Input: part model. Units: mm. Frame: model coordinates. A direction names the side the tool comes from. Give positions to 0.01 mm unless a question says otherwise; leave off trailing zeros. Order: outer loops, then holes, each group sorted by start corner. A loop starts at its lowest first (then second) coordinate and runs counter-clockwise, first axis right, second up. Notation, with made-up numbers: (6, -20) - (45, -20) arc R17 ccw to (45, -12) - close; hole circle Ø6 at (50, 14.25). An arc over 180 degrees is marked (long way). Use a Markdown table: item, result.
from build123d import *

# Parameters (mm, degrees)
SKETCH1_W                = 12.4
SKETCH1_H                = 5.75
BOSS_EXTRUDE1_DEPTH      = 7
SHELL1_T                 = -0.8
CUT_EXTRUDE1_DEPTH       = 13.4
CUT_EXTRUDE2_REACH       = 7.75
SKETCH4_W                = 0.64
SKETCH4_H                = 0.64
BOSS_EXTRUDE2_DEPTH      = 3.45
BOSS_EXTRUDE2_DEPTH_BACK = 6.75
CHAMFER1_SIZE            = 0.2


with BuildPart() as part:
    # Sketch1 → Boss-Extrude1 (new body)
    with BuildSketch(Plane(origin=(0, 0, 0), x_dir=(1, 0, 0), z_dir=(0, 1, 0))):
        Rectangle(SKETCH1_W, SKETCH1_H)
    extrude(amount=BOSS_EXTRUDE1_DEPTH)

    # Shell1
    shell1_openings = [part.faces().sort_by_distance(p)[0] for p in [
        (0, 7, 0),
    ]]
    offset(amount=SHELL1_T, openings=shell1_openings, kind=Kind.INTERSECTION)

    # Sketch2 → Cut-Extrude1 (cut, through all)
    with BuildSketch(Plane(origin=(6.2, 0, 0), x_dir=(0, 0, -1), z_dir=(1, 0, 0))):
        with BuildLine():
            Line((-1.19301282, 7), (-1.19301282, 4.379603984))
            ThreePointArc((-1.19301282, 4.379603984), (-1.72610374, 4.600417472), (-1.946917229, 5.133508392))
            Line((-1.946917229, 5.133508392), (-1.946917229, 7))
            Line((-1.946917229, 7), (-1.19301282, 7))
        make_face()
    extrude(amount=-CUT_EXTRUDE1_DEPTH, mode=Mode.SUBTRACT)

    # Sketch3 → Cut-Extrude2 (cut, up to next)
    with BuildSketch(Plane.XY.offset(2.875), mode=Mode.PRIVATE) as cut_extrude2_sk1:
        with BuildLine():
            Line((-4.2, 7), (-4.2, 6.728922615))
            Line((-4.2, 6.728922615), (-4.2, 5.166308225))
            ThreePointArc((-4.2, 5.166308225), (-3.946286554, 4.553789782), (-3.33376811, 4.300076336))
            Line((-3.33376811, 4.300076336), (-3.33376811, 7))
            Line((-3.33376811, 7), (-4.2, 7))
        make_face()
    cut_extrude2_tool1 = extrude(cut_extrude2_sk1.sketch, amount=-CUT_EXTRUDE2_REACH, mode=Mode.PRIVATE) & part.part
    add(cut_extrude2_tool1.solids().sort_by_distance((-3.749165, 5.735551, 2.875))[0], mode=Mode.SUBTRACT)
    # Sketch3 → Cut-Extrude2 (cut, up to next)
    with BuildSketch(Plane.XY.offset(2.875), mode=Mode.PRIVATE) as cut_extrude2_sk2:
        with BuildLine():
            Line((3.33376811, 7), (4.2, 7))
            Line((4.2, 7), (4.2, 6.728922615))
            Line((4.2, 6.728922615), (4.2, 5.166308225))
            ThreePointArc((4.2, 5.166308225), (3.946286554, 4.553789782), (3.33376811, 4.300076336))
            Line((3.33376811, 4.300076336), (3.33376811, 7))
        make_face()
    cut_extrude2_tool2 = extrude(cut_extrude2_sk2.sketch, amount=-CUT_EXTRUDE2_REACH, mode=Mode.PRIVATE) & part.part
    add(cut_extrude2_tool2.solids().sort_by_distance((3.749165, 5.735551, 2.875))[0], mode=Mode.SUBTRACT)

    # Sketch4 → Boss-Extrude2 (add, two sides)
    with BuildSketch(Plane.XZ) as boss_extrude2_sk:
        with Locations((-3.75, 0.525)):
            Rectangle(SKETCH4_W, SKETCH4_H)
        with Locations((-1.21, 0.525)):
            Rectangle(SKETCH4_W, SKETCH4_H)
        with Locations((1.33, 0.525)):
            Rectangle(SKETCH4_W, SKETCH4_H)
        with Locations((3.87, 0.525)):
            Rectangle(SKETCH4_W, SKETCH4_H)
    extrude(amount=BOSS_EXTRUDE2_DEPTH)
    extrude(boss_extrude2_sk.sketch, amount=-BOSS_EXTRUDE2_DEPTH_BACK)

    # Chamfer1
    chamfer1_edges = [part.edges().sort_by_distance(p)[0] for p in [
        (-1.21, 6.75, 0.205),
        (-1.53, 6.75, 0.525),
        (-1.21, 6.75, 0.845),
        (-0.89, 6.75, 0.525),
        (-1.21, -3.45, 0.205),
        (-0.89, -3.45, 0.525),
        (-1.21, -3.45, 0.845),
        (-1.53, -3.45, 0.525),
        (1.33, 6.75, 0.205),
        (1.01, 6.75, 0.525),
        (1.33, 6.75, 0.845),
        (1.65, 6.75, 0.525),
        (1.33, -3.45, 0.205),
        (1.65, -3.45, 0.525),
        (1.33, -3.45, 0.845),
        (1.01, -3.45, 0.525),
        (3.87, 6.75, 0.205),
        (3.55, 6.75, 0.525),
        (3.87, 6.75, 0.845),
        (4.19, 6.75, 0.525),
        (3.87, -3.45, 0.205),
        (4.19, -3.45, 0.525),
        (3.87, -3.45, 0.845),
        (3.55, -3.45, 0.525),
        (-3.43, 6.75, 0.525),
        (-3.75, 6.75, 0.205),
        (-4.07, 6.75, 0.525),
        (-3.75, 6.75, 0.845),
        (-3.43, -3.45, 0.525),
        (-3.75, -3.45, 0.845),
        (-4.07, -3.45, 0.525),
        (-3.75, -3.45, 0.205),
    ]]
    chamfer(chamfer1_edges, length=CHAMFER1_SIZE)


solid = part.part
1. Mould query, pull axis X, two halves, no side actions, for faces 4 (the face through (6.2, 3, 0)), 5 (the face through (0, 3, -2.875)), 6 (the face through (0, 4, 2.075)). Classes: pulls with the +X half, pulls with the -X half, needs draft (parallel to the pull), parting line crosses it, or undercut.
Response:
| item | result |
|---|---|
| face 4 | pulls with the +X half |
| face 5 | needs draft |
| face 6 | undercut |
2. Section query A-A (y = 2). Return loops of the section in (x, z) (3 decimals), then the cut area to 3 significant figures.
Response:
| item | result |
|---|---|
| outline | (-6.2, -2.875) - (6.2, -2.875) - (6.2, 2.875) - (-6.2, 2.875) - close; (-4.07, 0.205) - (-3.43, 0.205) - (-3.43, 0.845) - (-4.07, 0.845) - close; (-1.53, 0.205) - (-0.89, 0.205) - (-0.89, 0.845) - (-1.53, 0.845) - close; (1.01, 0.205) - (1.65, 0.205) - (1.65, 0.845) - (1.01, 0.845) - close; (3.55, 0.205) - (4.19, 0.205) - (4.19, 0.845) - (3.55, 0.845) - close; hole (-5.4, -2.075) - (5.4, -2.075) - (5.4, 2.075) - (-5.4, 2.075) - close |
| area | 28.1 mm^2 |
3. Material intervals for line 1 along Z through (x, y) = (-1, 1.5) (3 decimals); line 2 along X through (y, z) = (2.5, 0.75); line 3 along Z through (x, y) = (-2, 1) (3 decimals), sorted ascending.
Response:
| item | result |
|---|---|
| line 1 | z = -2.875 to -2.075, 0.205 to 0.845, 2.075 to 2.875 |
| line 2 | x = -6.2 to -5.4, -4.07 to -3.43, -1.53 to -0.89, 1.01 to 1.65, 3.55 to 4.19, 5.4 to 6.2 |
| line 3 | z = -2.875 to -2.075, 2.075 to 2.875 |
4. Pin query (flat end, axial travel): pin 1 (0.7 mm diameter, centred on x = 1.5, y = -1.5, fed in from -Z) (3 decimals); pin 2 (1.2 mm diameter, centred on x = -2.5, z = -0.5, fed in from +Y); pin 3 (1.5 mm diameter, centred on y = -2, z = -1.5, fed in from -X). Return the tip coordinate at first contact, or that it passes through.
Response:
| item | result |
|---|---|
| pin 1 | stops at z = 0.205 |
| pin 2 | stops at y = 0.8 |
| pin 3 | passes through |
5. Section query C-C (y = -1). Return loops of the section in (x, z) (3 decimals), then the cut area to 3 significant figures.
Response:
| item | result |
|---|---|
| outline | (-4.07, 0.205) - (-3.43, 0.205) - (-3.43, 0.845) - (-4.07, 0.845) - close; (-1.53, 0.205) - (-0.89, 0.205) - (-0.89, 0.845) - (-1.53, 0.845) - close; (1.01, 0.205) - (1.65, 0.205) - (1.65, 0.845) - (1.01, 0.845) - close; (3.55, 0.205) - (4.19, 0.205) - (4.19, 0.845) - (3.55, 0.845) - close |
| area | 1.64 mm^2 |
6. Section query B-B (z = 2.4). Return loops of the section in (x, y), then the cut area to 3 significant figures.
Response:
| item | result |
|---|---|
| outline | (-6.2, 0) - (6.2, 0) - (6.2, 7) - (4.2, 7) - (4.2, 5.17) arc R0.87 cw to (3.33, 4.3) - (3.33, 7) - (-3.33, 7) - (-3.33, 4.3) arc R0.87 cw to (-4.2, 5.17) - (-4.2, 7) - (-6.2, 7) - close |
| area | 82.4 mm^2 |
7. Section query D-D (x = 2). Return loops of the section in (y, z) (3 decimals), then the cut area to 3 significant figures.
Response:
| item | result |
|---|---|
| outline | (0, -2.875) - (7, -2.875) - (7, -2.075) - (0.8, -2.075) - (0.8, 2.075) - (7, 2.075) - (7, 2.875) - (0, 2.875) - close |
| area | 14.5 mm^2 |
8. Set-up query: faces 1 (the face through (-5.4, 4, 0)), 2 (the face through (0, 3, 2.875)), 3 (the face through (-3.95, 4.56, 2.48)). Return all of +Z, -Z, +X, -X, +Y, -Y with unobstructed straight access to the full face (end or side cutting, diameter ignored); none if empty.
Response:
| item | result |
|---|---|
| face 1 | +Y |
| face 2 | +Z, +X, -X, +Y, -Y |
| face 3 | +Z, +Y |
